Can you work these out from the model? Positions are in its coordinate system, mm. A direction names the side the tool comes from. Give positions to 0.01 mm unless a question says otherwise; leave off trailing zeros. Write each loop counter-clockwise with the first axis right and the second up, starting at its lowest first coordinate (ties: lowest second). Pieces come first, ordered by that corner, then holes.
```python
from build123d import *

# Parameters (mm, degrees)
F1_DEPTH = 5
F3_D     = 5.1
F4_R     = 2.55
F5_DEPTH = 25


with BuildPart() as f1:
    # F0 (on Top) → F1 (new body)
    with BuildSketch(Plane.XY):
        with BuildLine():
            Line((84.6812899327, 58.5268347502), (-92.3187100673, 58.5268347502))
            Line((-92.3187100673, 58.5268347502), (-92.3187100673, 8.5268347502))
            Line((-92.3187100673, 8.5268347502), (-92.3187100673, -51.4731652498))
            Line((-92.3187100673, -51.4731652498), (-54.3187100673, -51.4731652498))
            Line((-54.3187100673, -51.4731652498), (-54.3187100673, -1.4731652498))
            ThreePointArc((-54.3187100673, -1.4731652498), (-51.3897778791, 5.597902562), (-44.3187100673, 8.5268347502))
            Line((-44.3187100673, 8.5268347502), (36.6812899327, 8.5268347502))
            ThreePointArc((36.6812899327, 8.5268347502), (43.7523577446, 5.597902562), (46.6812899327, -1.4731652498))
            Line((46.6812899327, -1.4731652498), (46.6812899327, -51.4731652498))
            Line((46.6812899327, -51.4731652498), (84.6812899327, -51.4731652498))
            Line((84.6812899327, -51.4731652498), (84.6812899327, 8.5268347502))
            Line((84.6812899327, 8.5268347502), (84.6812899327, 58.5268347502))
        make_face()
    extrude(amount=F1_DEPTH)

    # F3 (through all)
    with Locations(Plane.XY.offset(5)):
        with Locations((-10.8187100673, 27.5268347502), (-3.8187100673, 48.5268347502), (3.1812899327, 27.5268347502), (-3.8187100673, 15.2268347502)):
            Hole(F3_D / 2)

    # F4 (on face) → F5 (cut)
    with BuildSketch(Plane.XY.offset(5)):
        Polygon((-79.3187100673, -16.7825663266), (-79.3187100673, -12.1637641731), (-83.3187100673, -9.8543630963), (-87.3187100673, -12.1637641731), (-87.3187100673, -16.7825663266), (-83.3187100673, -19.0919674033), align=None)
        Polygon((-69.3187100673, -46.2825663266), (-69.3187100673, -41.6637641731), (-73.3187100673, -39.3543630963), (-77.3187100673, -41.6637641731), (-77.3187100673, -46.2825663266), (-73.3187100673, -48.5919674033), align=None)
        Polygon((71.0691113787, -6.7204349793), (73.589342523, -10.5910639091), (78.201521077, -10.3437941797), (80.2934684868, -6.2258955204), (77.7732373424, -2.3552665905), (73.1610587884, -2.60253632), align=None)
        Polygon((70.3000901599, -43.9689468335), (67.9870367906, -39.9710577099), (63.3682365634, -39.9752761263), (61.0624897056, -43.9773836662), (63.3755430749, -47.9752727897), (67.994343302, -47.9710543734), align=None)
        with Locations((-63.3187100673, -6.4731652498)):
            Circle(F4_R)
        with Locations((55.6812899327, -14.4731652498)):
            Circle(F4_R)
    extrude(amount=-F5_DEPTH, mode=Mode.SUBTRACT)


solid = f1.part
```
1) Suppose I cut it at A-A on x = 20. Write out the boundary of the cut face in (y, z).
Values follow:
outline: (8.53, 0) - (58.53, 0) - (58.53, 5) - (8.53, 5) - close
2) Please list where these lines run through material, in increasing order: L1, parallel to X at y = 26, z = 2.95; L2, parallel to X at y = 50, z = 4.8; L3, parallel to X at y = 5, z = 1.25.
Values follow:
L1: x = -92.32 to -12.86, -8.78 to 1.14, 5.22 to 84.68
L2: x = -92.32 to -5.9, -1.74 to 84.68
L3: x = -92.32 to -51.94, 44.3 to 84.68
3) Suppose I cut it at B-B on z = 1.75. State how many separate pieces and enclosed holes the cut face has, plus the area to 3 significant figures.
Values follow:
separate pieces: 1
enclosed holes: 10
area: 13,100 mm2
4) If we mould it in two halves opening along Y, with no side actions, what happens to faces 1 (the face through (-51.467, 5.52, 2.465)), 2 (the face through (72.312, -8.629, 2.535)), 3 (the face through (84.681, 3, 2))? For each: +Y half, -Y half, draft (parallel to the pull), parting line (faces both ways), or undercut.
Values follow:
face 1: -Y half
face 2: undercut
face 3: draft
5) For faces 4 (the face through (-4, 8.527, 2)), 5 (the face through (-71.291, -40.525, 2.535)), which set-ups out of +Z, -Z, +X, -X, +Y, -Y let a thin tool reach every point of the face, with its end or its side?
Values follow:
face 4: +Z, -Z, -Y
face 5: +Z, -Z
6) Suppose I cut it at C-C on x = -47.5. Write out the boundary of the cut face in (y, z), plus the area to 3 significant figures.
Values follow:
outline: (8.01, 0) - (58.53, 0) - (58.53, 5) - (8.01, 5) - close
area: 253 mm2
7) For pin 1 Ø2.5 at (x, z) = (7.5, 1.5) entering from -Y, with a flat end and sliding along its axis, tell me the tip position at first contact or that it passes through.
Values follow:
pin 1: stops at y = 8.53
